Part print with two shaded views. Sizes in mm from the minimum x, y, z corner. Round coordinates to 2 decimals unless told otherwise and drop trailing zeros. Loops run counter-clockwise (first coordinate to the right, second up) from the corner with the lowest first, then second, coordinate; pieces in that order, holes last.
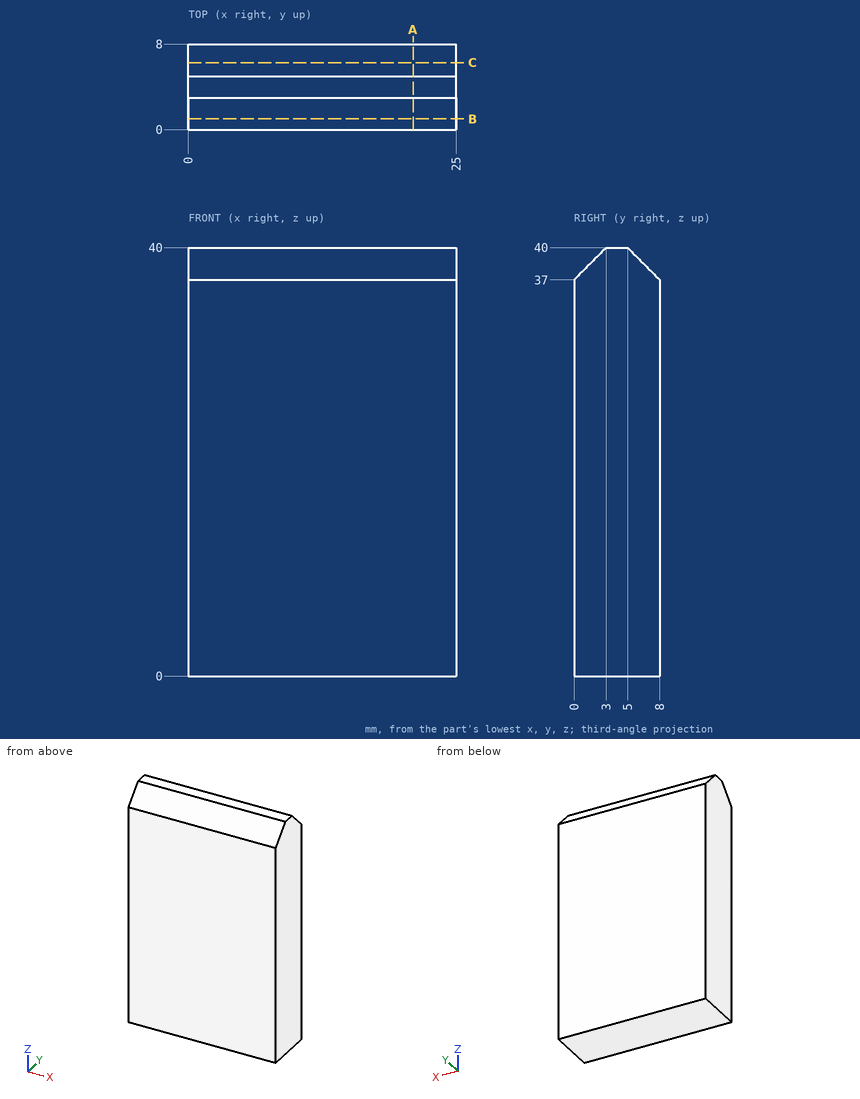
Item 1: Cut at C-C (y = 6.25). List the corners of the cut face in (x, z), plus the area to 3 significant figures.
Verdict:
outline: (0, 0) - (25, 0) - (25, 38.75) - (0, 38.75) - close
area: 969 mm2
Item 2: Flat gauge pin, fed straight in: P1, Ø2, axis at x = 15.5, y = 1, coming from the -Z side. Where does the tip first touch, or does it go through?
Verdict:
P1: stops at z = 0
Item 3: Wall check: L1, parallel to Z at x = 16, y = 1; L2, parallel to Z at x = 16, y = 5.25. Give the ranges that are in metal, low to high.
Verdict:
L1: z = 0 to 38
L2: z = 0 to 39.75
Item 4: Cut at B-B (y = 1). List the corners of the cut face in (x, z), plus the area to 3 significant figures.
Verdict:
outline: (0, 0) - (25, 0) - (25, 38) - (0, 38) - close
area: 950 mm2
Item 5: Cut at A-A (x = 21). List the corners of the cut face in (y, z), plus the area to 3 significant figures.
Verdict:
outline: (0, 0) - (8, 0) - (8, 37) - (5, 40) - (3, 40) - (0, 37) - close
area: 311 mm2
